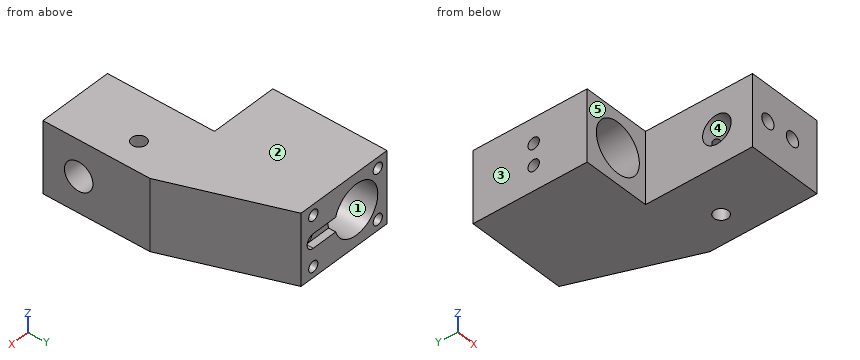
from build123d import *

# Parameters (mm, degrees)
BOSS_EXTRUDE1_DEPTH         = 20
SKETCH2_R                   = 7
CUT_EXTRUDE1_DEPTH          = 77.446059414
SKETCH3_R                   = 4
CUT_EXTRUDE2_DEPTH          = 55.990908339
SKETCH4_R                   = 2
CUT_EXTRUDE3_DEPTH          = 30
CUT_EXTRUDE5_DEPTH          = 2
SKETCH6_R                   = 2
CUT_EXTRUDE6_DEPTH          = 55.990908339
CUT_EXTRUDE7_REACH          = 56.991
CUT_EXTRUDE7_END_RADIUS     = 7
SKETCH7_R                   = 1.6
M3_TAPPED_HOLE1_D           = 2.5
M3_TAPPED_HOLE1_DEPTH       = 7.5
M3_TAPPED_HOLE1_CBORE_D     = 3
M3_TAPPED_HOLE1_CBORE_DEPTH = 6
M3_TAPPED_HOLE1_TIP         = 0.751075774
CUT_EXTRUDE8_START          = -20
SKETCH11_R                  = 2
CUT_EXTRUDE8_DEPTH          = 20
SKETCH12_R                  = 1.5
CUT_EXTRUDE9_DEPTH          = 12


with BuildPart() as part:
    # Sketch1 → Boss-Extrude1 (new body)
    with BuildSketch(Plane.XY):
        Polygon((0, 0), (0, -30), (-21, -30), (-21, 0), (-40, 0), (-40, 32), (-12, 32), align=None)
    extrude(amount=BOSS_EXTRUDE1_DEPTH)

    # Sketch2 → Cut-Extrude1 (cut, through all)
    with BuildSketch(Plane(origin=(0, 32, 0), x_dir=(1, 0, 0), z_dir=(0, 1, 0))):
        with Locations(Location((-30, -10, 0), (0, 0, 270))):
            Circle(SKETCH2_R)
    extrude(amount=-CUT_EXTRUDE1_DEPTH, mode=Mode.SUBTRACT)

    # Sketch3 → Cut-Extrude2 (cut, through all)
    with BuildSketch(Plane(origin=(0, 0, 0), x_dir=(0, 0, -1), z_dir=(1, 0, 0))):
        with Locations(Location((-10, -20, 0), (0, 0, 90))):
            Circle(SKETCH3_R)
    extrude(amount=-CUT_EXTRUDE2_DEPTH, mode=Mode.SUBTRACT)

    # Sketch4 → Cut-Extrude3 (cut)
    with BuildSketch(Plane(origin=(0, 32, 0), x_dir=(1, 0, 0), z_dir=(0, 1, 0))):
        with Locations(Location((-16, -10, 0), (0, 0, 270))):
            Circle(SKETCH4_R)
    extrude(amount=-CUT_EXTRUDE3_DEPTH, mode=Mode.SUBTRACT)

    # Sketch5 → Cut-Extrude5 (cut)
    with BuildSketch(Plane(origin=(0, 32, 0), x_dir=(1, 0, 0), z_dir=(0, 1, 0))):
        with BuildLine():
            Line((-16, -12), (-23.291796068, -12))
            ThreePointArc((-23.291796068, -12), (-23, -10), (-23.291796068, -8))
            Line((-23.291796068, -8), (-16, -8))
            ThreePointArc((-16, -8), (-14, -10), (-16, -12))
        make_face()
    extrude(amount=-CUT_EXTRUDE5_DEPTH, mode=Mode.SUBTRACT)

    # Sketch6 → Cut-Extrude6 (cut, through all)
    with BuildSketch(Plane.XY.offset(20)):
        with Locations((-8, -10)):
            Circle(SKETCH6_R)
    extrude(amount=-CUT_EXTRUDE6_DEPTH, mode=Mode.SUBTRACT)

    # Cut-Extrude7: up to this cylinder (the profile starts outside it)
    cut_extrude7_end = Plane(origin=(-30, 15, 10), z_dir=(0, 1, 0)) * Cylinder(CUT_EXTRUDE7_END_RADIUS, 128.982, mode=Mode.PRIVATE)
    # Sketch7 → Cut-Extrude7 (cut, up to the surface)
    with BuildSketch(Plane.ZY.offset(40), mode=Mode.PRIVATE) as cut_extrude7_sk1:
        with Locations((7, 15)):
            Circle(SKETCH7_R)
    cut_extrude7_tool1 = extrude(cut_extrude7_sk1.sketch, amount=-CUT_EXTRUDE7_REACH, mode=Mode.PRIVATE) - cut_extrude7_end
    add(cut_extrude7_tool1.solids().sort_by_distance((-40, 15, 7))[0], mode=Mode.SUBTRACT)
    # Sketch7 → Cut-Extrude7 (cut, up to the surface)
    with BuildSketch(Plane.ZY.offset(40), mode=Mode.PRIVATE) as cut_extrude7_sk2:
        with Locations((13, 15)):
            Circle(SKETCH7_R)
    cut_extrude7_tool2 = extrude(cut_extrude7_sk2.sketch, amount=-CUT_EXTRUDE7_REACH, mode=Mode.PRIVATE) - cut_extrude7_end
    add(cut_extrude7_tool2.solids().sort_by_distance((-40, 15, 13))[0], mode=Mode.SUBTRACT)

    # M3 Tapped Hole1
    with Locations(Plane(origin=(0, 32, 0), x_dir=(1, 0, 0), z_dir=(0, 1, 0))):
        with Locations((-37, -3), (-16, -3), (-16, -17), (-37, -17)):
            CounterBoreHole(M3_TAPPED_HOLE1_D / 2, M3_TAPPED_HOLE1_CBORE_D / 2, M3_TAPPED_HOLE1_CBORE_DEPTH, depth=M3_TAPPED_HOLE1_DEPTH)
            with Locations((0, 0, -(M3_TAPPED_HOLE1_DEPTH + M3_TAPPED_HOLE1_TIP / 2))):  # 118° drill point
                Cone(0, M3_TAPPED_HOLE1_D / 2, M3_TAPPED_HOLE1_TIP, mode=Mode.SUBTRACT)

    # Sketch11 → Cut-Extrude8 (cut)
    with BuildSketch(Plane.XZ.offset(30).offset(CUT_EXTRUDE8_START)):
        with Locations((-8, 10)):
            Circle(SKETCH11_R)
        with Locations(Location((-16, 10, 0), (0, 0, 90))):
            Circle(SKETCH11_R)
    extrude(amount=CUT_EXTRUDE8_DEPTH, mode=Mode.SUBTRACT)

    # Sketch12 → Cut-Extrude9 (cut)
    with BuildSketch(Plane(origin=(0, 2, 0), x_dir=(1, 0, 0), z_dir=(0, 1, 0))):
        with Locations(Location((-16, -10, 0), (0, 0, 270))):
            Circle(SKETCH12_R)
    extrude(amount=-CUT_EXTRUDE9_DEPTH, mode=Mode.SUBTRACT)


solid = part.part
Input: part model. Units: mm. Frame: model coordinates. Face numbers are marked on the shaded views. A direction names the side the tool comes from. Give positions to 0.01 mm unless a question says otherwise; leave off trailing zeros. Write each loop counter-clockwise with the first axis right and the second up, starting at its lowest first coordinate (ties: lowest second). Pieces come first, ordered by that corner, then holes. Notation, with made-up numbers: M 79.5,50 L 131.5,50 A11 cw 131.5,57 Z; hole C 57.5,84 d8. An arc over 180 degrees is marked long. Use one line per item in the form item = value.
1. Cut plane B-B on z = 6.75. Return loops of the section in (x, y).
Outcome:
outline = M -40,0 L -36.2,0 L -36.2,13.42 L -40,13.42 Z; M -40,16.58 L -36.2,16.58 L -36.2,32 L -40,32 Z; M -23.8,0 L -21,0 L -21,-17.67 L 0,-17.67 L 0,0 L -12,32 L -23.8,32 Z; M -21,-30 L 0,-30 L 0,-22.33 L -21,-22.33 Z; hole C -8,-10 d4
2. Cut plane D-D on y = 4. Return loops of the section in (x, z), and give its area (3 significant figures).
Outcome:
outline = M -40,0 L -1.5,0 L -1.5,20 L -40,20 Z; hole C -30,10 d14; hole C -16,10 d4
area = 603 mm²
3. Ray query, L1, parallel to X at y = -27.25, z = 10; L2, parallel to Z at x = -38.45, y = 15; L3, parallel to Z at x = -16, y = 27.9. Return the intervals inside material, ascending.
Outcome:
L1 = -21 to -18, -14 to -10, -6 to 0
L2 = 0 to 5.4, 8.6 to 11.4, 14.6 to 20
L3 = 0 to 1.5, 4.5 to 8, 12 to 15.5, 18.5 to 20
4. First-contact query: P1, Ø2, axis at x = -37, z = 3, coming from the -Y side; P2, Ø2.5, axis at x = -8, z = 10, coming from the -Y side; P3, Ø1.8, axis at x = -16, z = 3, coming from the +Y side. Flat tips, straight axial feed; report the tip coordinate or a pass-through.
Outcome:
P1 = 0
P2 = -8.44
P3 = 24.29
5. Mould query, pull axis X, two halves, no side actions, for the marked faces 1, 2 and 3. Classes: released by +X, released by -X, zero draft, split by the parting line, or undercut.
Outcome:
face_1 = undercut
face_2 = zero draft
face_3 = released by -X
6. Reachability of the marked faces 4 and 5 from +Z, -Z, +X, -X, +Y, -Y: full face, straight path, thin tool, end or side. Return the list, or none.
Outcome:
face_4 = +X, -X
face_5 = +Z, -Z, -X, -Y
7. Cut plane A-A on y = -20. Return loops of the section in (x, z), and give its area (3 significant figures).
Outcome:
outline = M -21,0 L 0,0 L 0,6 L -21,6 Z; M -21,14 L 0,14 L 0,20 L -21,20 Z
area = 252 mm²
8. Cut plane C-C on x = -25. Return loops of the section in (y, z).
Outcome:
outline = M 0,0 L 32,0 L 32,5.1 L 0,5.1 Z; M 0,14.9 L 32,14.9 L 32,20 L 0,20 Z
